from build123d import *

# Parameters (mm, degrees)
F0_R     = 29.21
F1_DEPTH = 31.75
F0_R_2   = 6.35
F2_DEPTH = 31.75
F3_DEPTH = 31.75


with BuildPart() as f1:
    # F0 (on Front) → F1 (new body)
    with BuildSketch(Plane.XZ):
        Circle(F0_R)
        with BuildLine():
            ThreePointArc((21.5331844423, 10.8893924428), (23.4718197057, 5.5973725715), (24.13, 0))
            ThreePointArc((24.13, 0), (17.4832992726, -16.6310296298), (1.2049153298, -24.0998979053))
            ThreePointArc((1.2049153298, -24.0998979053), (-0.0651750036, -24.1299119812), (-1.3350846702, -24.0930373536))
            ThreePointArc((-1.3350846702, -24.0930373536), (-21.1740501638, -11.5722296754), (-20.9990868902, 11.8867678441))
            ThreePointArc((-20.9990868902, 11.8867678441), (-20.3436941865, 12.9765560472), (-19.6317982914, 14.030302771))
            ThreePointArc((-19.6317982914, 14.030302771), (0.5669275044, 24.1233391802), (20.2692187002, 13.0925808489))
            ThreePointArc((20.2692187002, 13.0925808489), (20.9302111052, 12.0076293701), (21.5331844423, 10.8893924428))
        make_face(mode=Mode.SUBTRACT)
    extrude(amount=F1_DEPTH)



with BuildPart() as f2:
    # F0 (on Front) → F2 (new body)
    with BuildSketch(Plane.XZ):
        with BuildLine():
            ThreePointArc((8.89, 0), (8.7360592676, 1.6472305465), (8.2795683975, 3.2374136516))
            ThreePointArc((8.2795683975, 3.2374136516), (7.7321419682, 4.3870355119), (7.026094307, 5.4466594156))
            ThreePointArc((7.026094307, 5.4466594156), (0.5769925697, 8.8712558059), (-6.2613755065, 6.310885577))
            ThreePointArc((-6.2613755065, 6.310885577), (-7.1044258576, 5.3440839471), (-7.7995628745, 4.2660191005))
            ThreePointArc((-7.7995628745, 4.2660191005), (-7.9668054392, -3.9448841673), (-1.3350846702, -8.7891779435))
            ThreePointArc((-1.3350846702, -8.7891779435), (-0.0657591783, -8.8897567869), (1.2049153298, -8.8079667942))
            ThreePointArc((1.2049153298, -8.8079667942), (6.6986490161, -5.8446729044), (8.89, 0))
        make_face()
        Circle(F0_R_2, mode=Mode.SUBTRACT)
    extrude(amount=F2_DEPTH)


with BuildPart() as f1_1:
    add(f1.part)

    add(f2.part)  # F3 merges F2
    # F0 (on Front) → F3 (join)
    with BuildSketch(Plane.XZ):
        with BuildLine():
            Line((-6.2613755065, 6.310885577), (-19.6317982914, 14.030302771))
            ThreePointArc((-19.6317982914, 14.030302771), (-20.3436941865, 12.9765560472), (-20.9990868902, 11.8867678441))
            Line((-20.9990868902, 11.8867678441), (-7.7995628745, 4.2660191005))
            ThreePointArc((-7.7995628745, 4.2660191005), (-7.1044258576, 5.3440839471), (-6.2613755065, 6.310885577))
        make_face()
        with BuildLine():
            ThreePointArc((-1.3350846702, -24.0930373536), (-0.0651750036, -24.1299119812), (1.2049153298, -24.0998979053))
            Line((1.2049153298, -24.0998979053), (1.2049153298, -8.8079667942))
            ThreePointArc((1.2049153298, -8.8079667942), (-0.0657591783, -8.8897567869), (-1.3350846702, -8.7891779435))
            Line((-1.3350846702, -8.7891779435), (-1.3350846702, -24.0930373536))
        make_face()
        with BuildLine():
            Line((8.2795683975, 3.2374136516), (21.5331844423, 10.8893924428))
            ThreePointArc((21.5331844423, 10.8893924428), (20.9302111052, 12.0076293701), (20.2692187002, 13.0925808489))
            Line((20.2692187002, 13.0925808489), (7.026094307, 5.4466594156))
            ThreePointArc((7.026094307, 5.4466594156), (7.7321419682, 4.3870355119), (8.2795683975, 3.2374136516))
        make_face()
        with BuildLine():
            ThreePointArc((-20.9990868902, 11.8867678441), (-21.1740501638, -11.5722296754), (-1.3350846702, -24.0930373536))
            Line((-1.3350846702, -24.0930373536), (-1.3350846702, -8.7891779435))
            ThreePointArc((-1.3350846702, -8.7891779435), (-7.9668054392, -3.9448841673), (-7.7995628745, 4.2660191005))
            Line((-7.7995628745, 4.2660191005), (-20.9990868902, 11.8867678441))
        make_face()
        with BuildLine():
            Line((7.026094307, 5.4466594156), (20.2692187002, 13.0925808489))
            ThreePointArc((20.2692187002, 13.0925808489), (0.5669275044, 24.1233391802), (-19.6317982914, 14.030302771))
            Line((-19.6317982914, 14.030302771), (-6.2613755065, 6.310885577))
            ThreePointArc((-6.2613755065, 6.310885577), (0.5769925697, 8.8712558059), (7.026094307, 5.4466594156))
        make_face()
        with BuildLine():
            ThreePointArc((1.2049153298, -24.0998979053), (17.4832992726, -16.6310296298), (24.13, 0))
            ThreePointArc((24.13, 0), (23.4718197057, 5.5973725715), (21.5331844423, 10.8893924428))
            Line((21.5331844423, 10.8893924428), (8.2795683975, 3.2374136516))
            ThreePointArc((8.2795683975, 3.2374136516), (8.7360592676, 1.6472305465), (8.89, 0))
            ThreePointArc((8.89, 0), (6.6986490161, -5.8446729044), (1.2049153298, -8.8079667942))
            Line((1.2049153298, -8.8079667942), (1.2049153298, -24.0998979053))
        make_face()
    extrude(amount=F3_DEPTH)

    # F4: F1 across plane


with BuildPart() as f1_2:
    add(f1_1.part)
    add(f1_1.part.mirror(Plane.XZ))


solid = f1_2.part
Source: CAD feature listing. Evaluate the final solid. Frame: model axes, mm. Round coordinates to 2 decimals unless told otherwise and drop trailing zeros. Write each loop counter-clockwise with the first axis right and the second up, starting at its lowest first coordinate (ties: lowest second). Pieces come first, ordered by that corner, then holes. Notation, with made-up numbers: M 24,8.5 L 63,8.5 A13 ccw 63,12.5 Z; hole C 10.25,28 d9. An arc over 180 degrees is marked long. One line per item, written item: value. Start each with the question number.
Item 1: Section query B-B (z = 0). Return the cut outline in (x, y).
Item 2: Section query D-D (z = 24). Return the cut outline in (x, y), plus the area to 3 significant figures.
Item 3: Section query C-C (y = -25). Return the cut outline in (x, z), plus the area to 3 significant figures.
Item 4: Ray query, L1, parallel to Z at x = 0, y = 0.5; L2, parallel to Z at x = -19, y = 18.5; L3, parallel to Z at x = 1.5, y = -4.5. Return the intervals inside material, ascending. Write a range as from..to.
Item 5: Mould query, pull axis X, two halves, no side actions, for faces 1 (the cylindrical face through (-1.38, 0.44, -6.2)), 2 (the cylindrical face through (-21.53, -0.44, 19.74)), 3 (the flat face through (0, -31.75, 7)). Classes: pulls with the +X half, pulls with the -X half, needs draft (parallel to the pull), parting line crosses it, or undercut.
Item 6: Section query A-A (x = 0). Return the cut outline in (y, z), plus the area to 3 significant figures.
Item 7: Pin query (flat end, axial travel): pin 1 (12 mm diameter, centred on y = -19.5, z = -17.5, fed in from -X); pin 2 (1.5 mm diameter, centred on x = 3, z = 3.5, fed in from -Y); pin 3 (1 mm diameter, centred on y = -19, z = 9, fed in from -X); pin 4 (3 mm diameter, centred on y = 4.5, z = -14, fed in from +X). Return the tip coordinate at first contact, or that it passes through.
Result set:
1. outline: M -29.21,-31.75 L -6.35,-31.75 L -6.35,31.75 L -29.21,31.75 Z; M 6.35,-31.75 L 29.21,-31.75 L 29.21,31.75 L 6.35,31.75 Z
2. outline: M -16.65,-31.75 L 16.65,-31.75 L 16.65,31.75 L -16.65,31.75 Z
2. area: 2,110 mm²
3. outline: C 0,0 d58.42; hole C 0,0 d12.7
3. area: 2,550 mm²
4. L1: z = -29.21..-6.35, 6.35..29.21
4. L2: z = -22.19..22.19
4. L3: z = -29.17..-6.17, 6.17..29.17
5. face 1: undercut
5. face 2: parting line crosses it
5. face 3: needs draft
6. outline: M -31.75,-29.21 L 31.75,-29.21 L 31.75,-6.35 L -31.75,-6.35 Z; M -31.75,6.35 L 31.75,6.35 L 31.75,29.21 L -31.75,29.21 Z
6. area: 2,900 mm²
7. pin 1: stops at x = -26.85
7. pin 2: passes through
7. pin 3: stops at x = -27.95
7. pin 4: stops at x = 26.4
